```python
from build123d import *

# Parameters (mm, degrees)
ESQUISSE1_W      = 80
ESQUISSE1_H      = 40
ESQUISSE1_R      = 2.5
ESQUISSE1_R_2    = 1.1
EXTRUSION1_DEPTH = 3
CONG_1_R         = 2.5


with BuildPart() as part:
    # Esquisse1 → Extrusion1 (new body)
    with BuildSketch(Plane(origin=(0, 0, 0), x_dir=(1, 0, 0), z_dir=(0, 1, 0))):
        with Locations((40, 20)):
            Rectangle(ESQUISSE1_W, ESQUISSE1_H)
        with Locations((10, 10)):
            Circle(ESQUISSE1_R, mode=Mode.SUBTRACT)
        with Locations((70, 10)):
            Circle(ESQUISSE1_R, mode=Mode.SUBTRACT)
        with Locations((70, 30)):
            Circle(ESQUISSE1_R, mode=Mode.SUBTRACT)
        with Locations((10, 30)):
            Circle(ESQUISSE1_R, mode=Mode.SUBTRACT)
        with Locations((40, 28)):
            Circle(ESQUISSE1_R_2, mode=Mode.SUBTRACT)
        with Locations((48, 28)):
            Circle(ESQUISSE1_R_2, mode=Mode.SUBTRACT)
        with Locations((56, 28)):
            Circle(ESQUISSE1_R_2, mode=Mode.SUBTRACT)
        with Locations((40, 20)):
            Circle(ESQUISSE1_R_2, mode=Mode.SUBTRACT)
        with Locations((24, 12)):
            Circle(ESQUISSE1_R_2, mode=Mode.SUBTRACT)
        with Locations((56, 20)):
            Circle(ESQUISSE1_R_2, mode=Mode.SUBTRACT)
        with Locations((40, 12)):
            Circle(ESQUISSE1_R_2, mode=Mode.SUBTRACT)
        with Locations((48, 12)):
            Circle(ESQUISSE1_R_2, mode=Mode.SUBTRACT)
        with Locations((56, 12)):
            Circle(ESQUISSE1_R_2, mode=Mode.SUBTRACT)
        with Locations((32, 12)):
            Circle(ESQUISSE1_R_2, mode=Mode.SUBTRACT)
        with Locations((24, 20)):
            Circle(ESQUISSE1_R_2, mode=Mode.SUBTRACT)
        with Locations((24, 28)):
            Circle(ESQUISSE1_R_2, mode=Mode.SUBTRACT)
        with Locations((32, 28)):
            Circle(ESQUISSE1_R_2, mode=Mode.SUBTRACT)
    extrude(amount=EXTRUSION1_DEPTH)

    # Congé1
    cong_1_edges = [part.edges().sort_by_distance(p)[0] for p in [
        (0, 1.5, -40),
        (80, 1.5, -40),
        (80, 1.5, 0),
        (0, 1.5, 0),
    ]]
    fillet(cong_1_edges, radius=CONG_1_R)


solid = part.part
```
Check sheet for the modelled part. Datum: model origin and axes. Units: mm. Round coordinates to 2 decimals unless told otherwise and drop trailing zeros. Loops run counter-clockwise (first coordinate to the right, second up) from the corner with the lowest first, then second, coordinate; pieces in that order, holes last. Notation, with made-up numbers: M -31.75,-2 L -9.75,-2 A20 ccw -9.75,16 Z; hole C 87,-18.75 d3. An arc over 180 degrees is marked long. Answer as a JSON object with one key per item and string values.
1. Section check B-B (x = 24). Record the boundary of the cut face in (y, z), plus the area to 3 significant figures.
Reply:
{"outline": "M 0,-40 L 3,-40 L 3,-29.1 L 0,-29.1 Z; M 0,-26.9 L 3,-26.9 L 3,-21.1 L 0,-21.1 Z; M 0,-18.9 L 3,-18.9 L 3,-13.1 L 0,-13.1 Z; M 0,-10.9 L 3,-10.9 L 3,0 L 0,0 Z", "area": "100 mm²"}
2. Section check C-C (y = 1.05). State how many separate pieces and enclosed holes the cut face has, plus the area to 3 significant figures.
Reply:
{"separate pieces": "1", "enclosed holes": "17", "area": "3,070 mm²"}
3. Section check A-A (z = -20). Record the boundary of the cut face in (x, y), plus the area to 3 significant figures.
Reply:
{"outline": "M 0,0 L 22.9,0 L 22.9,3 L 0,3 Z; M 25.1,0 L 38.9,0 L 38.9,3 L 25.1,3 Z; M 41.1,0 L 54.9,0 L 54.9,3 L 41.1,3 Z; M 57.1,0 L 80,0 L 80,3 L 57.1,3 Z", "area": "220 mm²"}
4. Scan lines: line 1 (Z direction, x = 10, y = 1.8); line 2 (Z direction, x = 48, y = 1.05); line 3 (Z direction, x = 24, y = 1.65). Record each from-to range of solid material in increasing order.
Reply:
{"line 1": "z = -40 to -32.5, -27.5 to -12.5, -7.5 to 0", "line 2": "z = -40 to -29.1, -26.9 to -13.1, -10.9 to 0", "line 3": "z = -40 to -29.1, -26.9 to -21.1, -18.9 to -13.1, -10.9 to 0"}
5. Mould release check, pull along X, two halves, no side actions. Record for faces 1 (the cylindrical face through (55.13, 1.48, -27.33)), 2 (the cylindrical face through (0.713, 1.521, -0.752)), 3 (the flat face through (39, 1, -40)): pulls with the +X half, pulls with the -X half, needs draft (parallel to the pull), parting line crosses it, or undercut.
Reply:
{"face 1": "undercut", "face 2": "pulls with the -X half", "face 3": "needs draft"}
6. Gauge pin test, flat end, axial feed: P1, Ø1.8, axis at x = 32, z = -12, coming from the +Y side. Record the tip position at first contact, or that the pin passes through.
Reply:
{"P1": "passes through"}
7. Section check D-D (x = 48). Record the boundary of the cut face in (y, z).
Reply:
{"outline": "M 0,-40 L 3,-40 L 3,-29.1 L 0,-29.1 Z; M 0,-26.9 L 3,-26.9 L 3,-13.1 L 0,-13.1 Z; M 0,-10.9 L 3,-10.9 L 3,0 L 0,0 Z"}
